from build123d import *

# Parameters (mm, degrees)
SKETCH1_R           = 2.75
SKETCH1_R_2         = 2.5
BOSS_EXTRUDE2_DEPTH = 5


with BuildPart() as part:
    # Sketch1 → Boss-Extrude2 (new body)
    with BuildSketch(Plane(origin=(0, 0, 0), x_dir=(1, 0, 0), z_dir=(0, 1, 0))):
        Polygon((135.199443114, 0), (0, 0), (-79.800556886, 110), (-79.800556886, 148.75), (135.199443114, 148.75), align=None)
        with Locations(Location((15.199443114, 10, 0), (0, 0, 270))):
            Circle(SKETCH1_R, mode=Mode.SUBTRACT)
        with Locations(Location((47.199443114, 10, 0), (0, 0, 270))):
            Circle(SKETCH1_R, mode=Mode.SUBTRACT)
        with Locations(Location((15.199443114, 120, 0), (0, 0, 270))):
            Circle(SKETCH1_R, mode=Mode.SUBTRACT)
        with Locations(Location((47.199443114, 120, 0), (0, 0, 270))):
            Circle(SKETCH1_R, mode=Mode.SUBTRACT)
        with Locations(Location((-55.300556886, 133.75, 0), (0, 0, 270))):
            Circle(SKETCH1_R_2, mode=Mode.SUBTRACT)
        with Locations(Location((97.699443114, 133.75, 0), (0, 0, 270))):
            Circle(SKETCH1_R_2, mode=Mode.SUBTRACT)
        Polygon((20.199443114, 102.925904836), (108.125347951, 20), (20.199443114, 20), align=None, mode=Mode.SUBTRACT)
        Polygon((27.273538278, 110), (115.199443114, 27.074095164), (115.199443114, 110), align=None, mode=Mode.SUBTRACT)
        Polygon((-55.091921611, 110), (10.199443114, 20), (10.199443114, 110), align=None, mode=Mode.SUBTRACT)
    extrude(amount=BOSS_EXTRUDE2_DEPTH)


solid = part.part
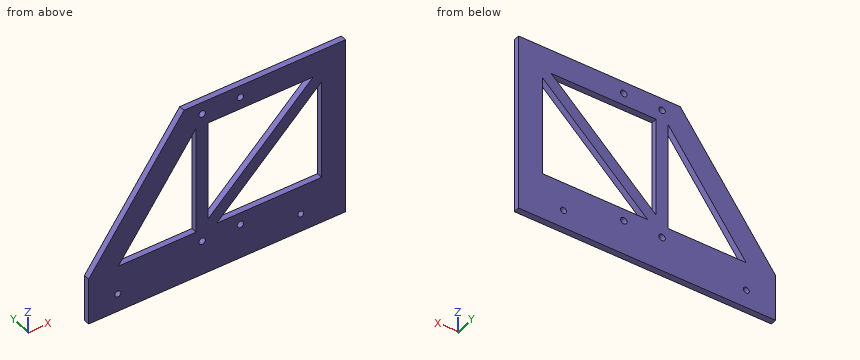
The model under review builds one solid part; all positions refer to its coordinate system, in mm. Round coordinates to 2 decimals unless told otherwise and drop trailing zeros. Write each loop counter-clockwise with the first axis right and the second up, starting at its lowest first coordinate (ties: lowest second). Pieces come first, ordered by that corner, then holes. Notation, with made-up numbers: M 80.5,61 L 100.5,61 A26 cw 100.5,95 Z; hole C -13,11.25 d1. An arc over 180 degrees is marked long. Use a Markdown table: item, result. Add a question column.
Q1. We need section C-C, the plane x = -47. State the section outline as (y, z) points, plus the area to 3 significant figures.
Q2. To check wall thickness, follow line 1 (X direction, y = 2.5, z = -10); line 2 (X direction, y = 2.15, z = -133.75); line 3 (X direction, y = 1.1, z = -83.5). State the ranges of each line that lie inside material, in increasing order.
Q3. Insertion check: pin 1 (5 mm diameter, centred on x = 47.2, z = -10, fed in from -Y); pin 2 (10 mm diameter, centred on x = 112.5, z = -82.5, fed in from +Y); pin 3 (2 mm diameter, centred on x = -43.5, y = 3.5, fed in from +Z); pin 4 (1.5 mm diameter, centred on x = -35.5, y = 3.5, fed in from +Z). Each pin has a flat end and moves straight along its axis. Give the tip position at first contact, or say it passes through.
Q4. We need section D-D, the plane x = 70.5. State the section outline as (y, z) points, plus the area to 3 significant figures.
Q5. We need section A-A, the plane z = -133.75. State the section outline as (x, y) points, plus the area to 4 significant figures.
Q6. We need section B-B, the plane z = -66.5. State the section outline as (x, y) points.
Findings below:
| question | item | result |
|---|---|---|
| 1 | outline | M 0,-148.75 L 5,-148.75 L 5,-110 L 0,-110 Z; M 0,-98.85 L 5,-98.85 L 5,-64.79 L 0,-64.79 Z |
| 1 | area | 364 mm² |
| 2 | line 1 | x = -7.25 to 12.45, 17.95 to 44.45, 49.95 to 135.2 |
| 2 | line 2 | x = -79.8 to -57.8, -52.8 to 95.2, 100.2 to 135.2 |
| 2 | line 3 | x = -60.58 to -35.87, 10.2 to 20.2, 40.8 to 55.37, 115.2 to 135.2 |
| 3 | pin 1 | passes through |
| 3 | pin 2 | stops at y = 5 |
| 3 | pin 3 | stops at z = -58.58 |
| 3 | pin 4 | stops at z = -47.9 |
| 4 | outline | M 0,-148.75 L 5,-148.75 L 5,-110 L 0,-110 Z; M 0,-69.23 L 5,-69.23 L 5,-55.49 L 0,-55.49 Z; M 0,-20 L 5,-20 L 5,0 L 0,0 Z |
| 4 | area | 362 mm² |
| 5 | outline | M -79.8,0 L -57.8,0 L -57.8,5 L -79.8,5 Z; M -52.8,0 L 95.2,0 L 95.2,5 L -52.8,5 Z; M 100.2,0 L 135.2,0 L 135.2,5 L 100.2,5 Z |
| 5 | area | 1,025 mm² |
| 6 | outline | M -48.24,0 L -23.53,0 L -23.53,5 L -48.24,5 Z; M 10.2,0 L 20.2,0 L 20.2,5 L 10.2,5 Z; M 58.82,0 L 73.4,0 L 73.4,5 L 58.82,5 Z; M 115.2,0 L 135.2,0 L 135.2,5 L 115.2,5 Z |
